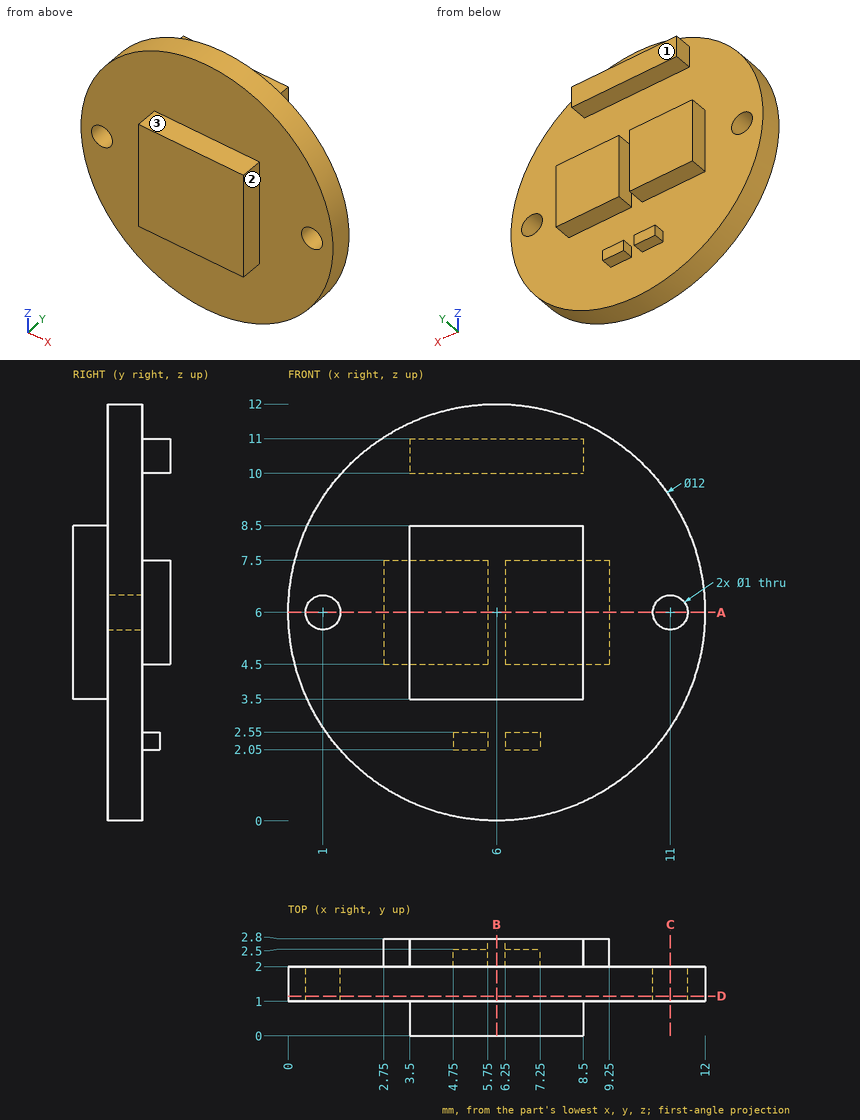
Geometry: see drawing. Coordinates: mm, zero at the bounding-box minimum. A direction names the side the tool comes from. Coordinates: 2 decimals unless noted, no trailing zeros. Write each loop counter-clockwise with the first axis right and the second up, starting at its lowest first coordinate (ties: lowest second). Pieces come first, ordered by that corner, then holes. Notation, with made-up numbers: (-38, 38) - (-12, 38) arc R31 cw to (-12, 70) - close; hole circle Ø8 at (-36.5, -34). An arc over 180 degrees is marked (long way). Put each result on its own line as item: value. Start each with the question number.
1) Cut plane C-C (x = 11). Return the cut outline in (y, z), plus the area to 3 significant figures.
2) Cut plane B-B (x = 6). Return the cut outline in (y, z), plus the area to 3 significant figures.
3) Ray query, L1, parallel to X at y = 1.45, z = 6; L2, parallel to X at y = 1.15, z = 5.75; L3, parallel to Y at x = 3.25, z = 1.25. Return the intervals inside material, ascending.
4) Reachability of the marked faces 1, 2 and 3 from +Z, -Z, +X, -X, +Y, -Y: full face, straight path, thin tool, end or side. Return the list, or none.
5) Cut plane A-A (z = 6). Return the cut outline in (x, y).
6) Cut plane D-D (y = 1.15). Return the cut outline in (x, z), plus the area to 3 significant figures.
7) Contact query for flat-ended pins moving along their axis: pin 1 (1.1 mm diameter, centred on x = 5.5, y = 0.5, fed in from +Z); pin 2 (0.6 mm diameter, centred on x = 7, y = 2.5, fed in from -Z); pin 3 (0.8 mm diameter, centred on y = 0.5, z = 5, fed in from -X). Output: stop coordinate, or through.
Resolved:
1. outline: (1, 2.68) - (2, 2.68) - (2, 5.5) - (1, 5.5) - close; (1, 6.5) - (2, 6.5) - (2, 9.32) - (1, 9.32) - close
1. area: 5.63 mm2
2. outline: (0, 3.5) - (1, 3.5) - (1, 0) - (2, 0) - (2, 10) - (2.8, 10) - (2.8, 11) - (2, 11) - (2, 12) - (1, 12) - (1, 8.5) - (0, 8.5) - close
2. area: 17.8 mm2
3. L1: x = 0 to 0.5, 1.5 to 10.5, 11.5 to 12
3. L2: x = 0.01 to 0.57, 1.43 to 10.57, 11.43 to 11.99
3. L3: y = 1 to 2
4. face 1: +Z, -Z, +X, -X, +Y
4. face 2: +Z, -Z, +X, -Y
4. face 3: +Z, +X, -X, -Y
5. outline: (0, 1) - (0.5, 1) - (0.5, 2) - (0, 2) - close; (1.5, 1) - (3.5, 1) - (3.5, 0) - (8.5, 0) - (8.5, 1) - (10.5, 1) - (10.5, 2) - (9.25, 2) - (9.25, 2.8) - (6.25, 2.8) - (6.25, 2) - (5.75, 2) - (5.75, 2.8) - (2.75, 2.8) - (2.75, 2) - (1.5, 2) - close; (11.5, 1) - (12, 1) - (12, 2) - (11.5, 2) - close
6. outline: circle Ø12 at (6, 6); hole circle Ø1 at (1, 6); hole circle Ø1 at (11, 6)
6. area: 112 mm2
7. pin 1: stops at z = 11.99
7. pin 2: stops at z = 2.05
7. pin 3: stops at x = 3.5
